Read the model definition and answer for the solid it produces. Units are mm, in the model's axes. Face numbers are marked on the shaded views. A direction names the side the tool comes from. Give positions to 0.01 mm unless a question says otherwise; leave off trailing zeros. Write each loop counter-clockwise with the first axis right and the second up, starting at its lowest first coordinate (ties: lowest second). Pieces come first, ordered by that corner, then holes. Notation, with made-up numbers: M 12.5,81.25 L 29.5,81.25 A14 cw 29.5,92.25 Z; hole C 80,-39.5 d3. An arc over 180 degrees is marked long. Use a Markdown table: item, result. Add a question column.
Item 1: A cutting plane is placed at A-A on y = -8. Determine the outline of the cut face in (x, z), then the cut area to 3 significant figures.
Item 2: A cutting plane is placed at C-C on z = 9.5. Determine the outline of the cut face in (x, y), then the cut area to 3 significant figures.
Item 3: Consider probe 1 along Y at (x, z) = (96.5, 15); probe 2 along X at (y, z) = (17.5, -16.5). Determine where each line is inside the solid, lowest interval first. Write a range as [from, to].
Item 4: The mould has two halves that part along Y. Classify the marked faces 1, 2 and 3: pulls with the +Y half, pulls with the -Y half, needs draft (parallel to the pull), parting line crosses it, or undercut.
Item 5: For the marked faces 4 and 5, determine the directions among +Z, -Z, +X, -X, +Y, -Y from which every point of the face is accessible in a straight line to the end or side of a thin tool.
Item 6: A cutting plane is placed at B-B on x = 55.5. Determine the outline of the cut face in (y, z) (3 decimals).
from build123d import *

# Parameters (mm, degrees)
EXTRUDE_THIN1_DEPTH     = 123.98756
CUT_EXTRUDE1_DEPTH      = 1
CUT_EXTRUDE1_DEPTH_BACK = 39.1
CUT_EXTRUDE2_DEPTH      = 1
CUT_EXTRUDE2_DEPTH_BACK = 39.1


with BuildPart() as part:
    # Sketch1 → Extrude-Thin1 (new body, symmetric)
    with BuildSketch(Plane(origin=(0, 0, 0), x_dir=(0, 0, -1), z_dir=(1, 0, 0))):
        with BuildLine():
            Line((-15.875, 19.05), (15.875, 19.05))
            ThreePointArc((15.875, 19.05), (18.12006403, 18.12006403), (19.05, 15.875))
            Line((19.05, 15.875), (19.05, -15.875))
            ThreePointArc((19.05, -15.875), (18.12006403, -18.12006403), (15.875, -19.05))
            Line((15.875, -19.05), (-15.875, -19.05))
            ThreePointArc((-15.875, -19.05), (-18.12006403, -18.12006403), (-19.05, -15.875))
            Line((-19.05, -15.875), (-19.05, 15.875))
            ThreePointArc((-19.05, 15.875), (-18.12006403, 18.12006403), (-15.875, 19.05))
        make_face()
        with BuildLine():
            Line((-15.875, 16.51), (15.875, 16.51))
            ThreePointArc((15.875, 16.51), (16.324012806, 16.324012806), (16.51, 15.875))
            Line((16.51, 15.875), (16.51, -15.875))
            ThreePointArc((16.51, -15.875), (16.324012806, -16.324012806), (15.875, -16.51))
            Line((15.875, -16.51), (-15.875, -16.51))
            ThreePointArc((-15.875, -16.51), (-16.324012806, -16.324012806), (-16.51, -15.875))
            Line((-16.51, -15.875), (-16.51, 15.875))
            ThreePointArc((-16.51, 15.875), (-16.324012806, 16.324012806), (-15.875, 16.51))
        make_face(mode=Mode.SUBTRACT)
    extrude(amount=EXTRUDE_THIN1_DEPTH, both=True)

    # Sketch3 → Cut-Extrude1 (cut, two sides)
    with BuildSketch(Plane(origin=(0, 19.05, 0), x_dir=(1, 0, 0), z_dir=(0, 1, 0))) as cut_extrude1_sk:
        Polygon((299.02319091, -499.956443526), (123.98756, -19.05), (110.120294074, 19.05), (-64.915336836, 499.956443526), (896.897550216, 850.027705346), (1260.836077962, -149.885181705), align=None)
    extrude(amount=CUT_EXTRUDE1_DEPTH, mode=Mode.SUBTRACT)
    extrude(cut_extrude1_sk.sketch, amount=-CUT_EXTRUDE1_DEPTH_BACK, mode=Mode.SUBTRACT)

    # Sketch4 → Cut-Extrude2 (cut, two sides)
    with BuildSketch(Plane(origin=(0, 19.05, 0), x_dir=(1, 0, 0), z_dir=(0, 1, 0))) as cut_extrude2_sk:
        Polygon((-516.026084699, -348.009381482), (-123.98756, -19.05), (-78.581748122, 19.05), (313.456776576, 348.009381482), (-344.461986387, 1132.086430879), (-1173.944847663, 436.067667915), align=None)
    extrude(amount=CUT_EXTRUDE2_DEPTH, mode=Mode.SUBTRACT)
    extrude(cut_extrude2_sk.sketch, amount=-CUT_EXTRUDE2_DEPTH_BACK, mode=Mode.SUBTRACT)


solid = part.part
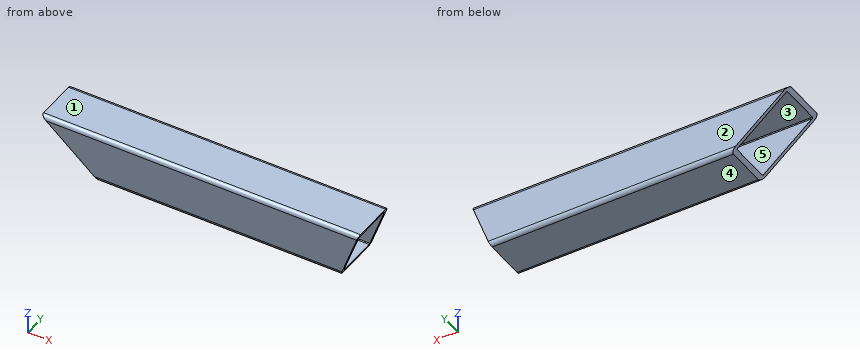
Filled in:
| question | item | result |
|---|---|---|
| 1 | outline | M -123.99,19.05 L -120.96,16.51 L 123.06,16.51 L 123.99,19.05 Z; M -81.61,-16.51 L -78.58,-19.05 L 110.12,-19.05 L 111.04,-16.51 Z |
| 1 | area | 1,110 mm² |
| 2 | outline | M -112.61,-19.05 L 120.51,-19.05 L 120.51,-16.51 L -112.61,-16.51 Z; M -112.61,16.51 L 120.51,16.51 L 120.51,19.05 L -112.61,19.05 Z |
| 2 | area | 1,180 mm² |
| 3 | probe 1 | [-19.05, -16.51], [16.51, 19.05] |
| 3 | probe 2 | [-81.62, 111.05] |
| 4 | face 1 | needs draft |
| 4 | face 2 | pulls with the +Y half |
| 4 | face 3 | undercut |
| 5 | face 4 | -Z, +X, -X, +Y, -Y |
| 5 | face 5 | +X, -X |
| 6 | outline | M -19.05,-15.875 A3.175 ccw -15.875,-19.05 L 15.875,-19.05 A3.175 ccw 19.05,-15.875 L 19.05,15.875 A3.175 ccw 15.875,19.05 L -15.875,19.05 A3.175 ccw -19.05,15.875 Z; hole M -16.51,-15.875 A0.635 ccw -15.875,-16.51 L 15.875,-16.51 A0.635 ccw 16.51,-15.875 L 16.51,15.875 A0.635 ccw 15.875,16.51 L -15.875,16.51 A0.635 ccw -16.51,15.875 Z |
